```python
from build123d import *

# Parameters (mm, degrees)
BOSS_EXTRUDE1_DEPTH   = 5
F_3_0MM_DOWEL_HOLE1_D = 3


with BuildPart() as part:
    # Sketch2 → Revolve1 (revolve)
    with BuildSketch(Plane(origin=(0, 0, 0), x_dir=(1, 0, 0), z_dir=(0, 1, 0))):
        with BuildLine():
            Line((29.047375097, 0), (29.047375097, 7.5))
            ThreePointArc((29.047375097, 7.5), (0, 30), (-29.047375097, 7.5))
            Line((-29.047375097, 7.5), (-29.047375097, 0))
            Line((-29.047375097, 0), (29.047375097, 0))
        make_face()
    revolve(axis=Axis((-29.047375097, 0, 0), (1, 0, 0)))

    # Sketch3 → Boss-Extrude1 (add)
    with BuildSketch(Plane.ZY.offset(29.047375097)):
        with BuildLine():
            Line((-7.5, 0), (-7.5, 70))
            Line((-7.5, 70), (7.5, 70))
            Line((7.5, 70), (7.5, 0))
            ThreePointArc((7.5, 0), (0, -7.5), (-7.5, 0))
        make_face()
    boss_extrude1 = extrude(amount=-BOSS_EXTRUDE1_DEPTH)

    # Mirror1: Boss-Extrude1 across plane
    add(boss_extrude1.mirror(Plane(origin=(0, 0, 0), x_dir=(0, 0, 1), z_dir=(1, 0, 0))))

    # Ø3.0mm Dowel Hole1 (through all)
    with Locations(Plane.ZY.offset(29.047375097)):
        with Locations((0, 60), (0, 40)):
            Hole(F_3_0MM_DOWEL_HOLE1_D / 2)


solid = part.part
```
Design review of the part built by this model. Coordinates are the model's own, in mm. A direction names the side the tool comes from. Give positions to 0.01 mm unless a question says otherwise; leave off trailing zeros. Loops run counter-clockwise (first coordinate to the right, second up) from the corner with the lowest first, then second, coordinate; pieces in that order, holes last. Notation, with made-up numbers: (71, -24) -> (90, -24) arc R21 ccw to (90, -19) -> close; hole circle Ø5 at (9.5, -29.75). An arc over 180 degrees is marked (long way). One line per item, written item: value.
Q1. Draft analysis for pull direction Y (two halves, no side actions). For faces 1 (the flat face through (-27, 70, 0)), 2 (the cylindrical face through (26.582, 38.536, 0.325)), 3 (the flat face through (27, 43, 7.5)), state which applies: pulls with the +Y half, pulls with the -Y half, needs draft (parallel to the pull), parting line crosses it, or undercut.
Numbers:
face 1: pulls with the +Y half
face 2: undercut
face 3: needs draft
Q2. For L1, parallel to X at y = 35, z = 0.5; L2, parallel to Y at x = 26.45, z = 0; L3, parallel to X at y = 21, z = 5.5, list the stretches that pass through material, from the lowest coordinate up.
Numbers:
L1: x = -29.05 to -24.05, 24.05 to 29.05
L2: y = -14.16 to 38.5, 41.5 to 58.5, 61.5 to 70
L3: x = -29.05 to -24.05, -20.71 to 20.71, 24.05 to 29.05
Q3. We need section A-A on y = 60. Give the boundary of the cut face in (x, z), and give its area (3 significant figures).
Numbers:
outline: (-29.05, -7.5) -> (-24.05, -7.5) -> (-24.05, -1.5) -> (-29.05, -1.5) -> close; (-29.05, 1.5) -> (-24.05, 1.5) -> (-24.05, 7.5) -> (-29.05, 7.5) -> close; (24.05, -7.5) -> (29.05, -7.5) -> (29.05, -1.5) -> (24.05, -1.5) -> close; (24.05, 1.5) -> (29.05, 1.5) -> (29.05, 7.5) -> (24.05, 7.5) -> close
area: 120 mm^2
Q4. We need section B-B on y = 33. Give the boundary of the cut face in (x, z).
Numbers:
outline: (-29.05, -7.5) -> (-24.05, -7.5) -> (-24.05, 7.5) -> (-29.05, 7.5) -> close; (24.05, -7.5) -> (29.05, -7.5) -> (29.05, 7.5) -> (24.05, 7.5) -> close
Q5. We need section C-C on z = 0. Give the boundary of the cut face in (x, y), and give its area (3 significant figures).
Numbers:
outline: (-29.05, -7.5) arc R30 ccw to (29.05, -7.5) -> (29.05, 38.5) -> (24.05, 38.5) -> (24.05, 17.94) arc R30 ccw to (-24.05, 17.94) -> (-24.05, 38.5) -> (-29.05, 38.5) -> close; (-29.05, 41.5) -> (-24.05, 41.5) -> (-24.05, 58.5) -> (-29.05, 58.5) -> close; (-29.05, 61.5) -> (-24.05, 61.5) -> (-24.05, 70) -> (-29.05, 70) -> close; (24.05, 41.5) -> (29.05, 41.5) -> (29.05, 58.5) -> (24.05, 58.5) -> close; (24.05, 61.5) -> (29.05, 61.5) -> (29.05, 70) -> (24.05, 70) -> close
area: 3,310 mm^2
Q6. We need section D-D on y = 19.5. Give the boundary of the cut face in (x, z).
Numbers:
outline: (-29.05, -7.5) -> (-24.05, -7.5) -> (-24.05, 7.5) -> (-29.05, 7.5) -> close; circle Ø45.6 at (0, 0); (24.05, -7.5) -> (29.05, -7.5) -> (29.05, 7.5) -> (24.05, 7.5) -> close
Q7. Machinability: for faces 4 (the flat face through (-27, 42, -7.5)), 5 (the flat face through (27, 42, -7.5)), 6 (the flat face through (-27, 43, 7.5)), which of the approach directions +Z, -Z, +X, -X, +Y, -Y give a long, thin tool a straight path to every point of the face, cutting with its end or side? Answer none if there is none.
Numbers:
face 4: -Z, -X, +Y
face 5: -Z, +X, +Y
face 6: +Z, -X, +Y
Q8. For pin 1 Ø1 at (x, z) = (-5.5, -22) entering from -Y; pin 2 Ø1.8 at (y, z) = (60, 0) entering from +X; pin 3 Ø1.5 at (x, y) = (27, 42.5) entering from +Z; pin 4 Ø4.5 at (y, z) = (39.5, -1) entering from +X, all flat-tipped, find the tip position at first contact; note any pin that passes through.
Numbers:
pin 1: stops at y = -20.2
pin 2: passes through
pin 3: stops at z = 7.5
pin 4: stops at x = 29.05
